The figure shows three views and two pictorial views of one solid part (mm, origin at its lowest corner). Answer the questions. Round coordinates to 2 decimals unless told otherwise and drop trailing zeros. Loops run counter-clockwise (first coordinate to the right, second up) from the corner with the lowest first, then second, coordinate; pieces in that order, holes last. Notation, with made-up numbers: (40.5, 47.25) -> (91.5, 47.25) arc R28 cw to (91.5, 69.25) -> close; hole circle Ø8 at (73.25, 42). An arc over 180 degrees is marked (long way). Use a Markdown table: item, result. Add a question column.
Q1. For a pull along X with two mould halves and no side action, classify the marked faces 1, 2 and 3 as released by +X, released by -X, zero draft, split by the parting line, or undercut.
Q2. Section B-B on z = 2.05 is taken. Give the vertices of the cut face in (x, y).
Q3. Given pin 1 Ø5 at (x, y) = (37.5, 49) entering from -Z; pin 2 Ø12.5 at (x, y) = (38.5, 35.5) entering from +Z; pin 3 Ø12 at (x, y) = (57, 33) entering from +Z; pin 4 Ø1.5 at (y, z) = (47, 1) entering from -X (1 decimal), each flat-ended and moving along its own axis, determine where each tip first touches the part or whether it passes through.
Q4. Consider line 1 (Y direction, x = 40, z = 2.15); line 2 (Y direction, x = 17.5, z = 5.5) (1 decimal); line 3 (X direction, y = 33.5, z = 0.5). Determine where each line is inside the solid, lowest interval first.
Q5. Section A-A on x = 40 is taken. Give the vertices of the cut face in (y, z).
Q6. Section D-D on y = 9 is taken. Give the vertices of the cut face in (x, z) (1 decimal).
Q7. Section C-C on y = 40 is taken. Give the vertices of the cut face in (x, z).
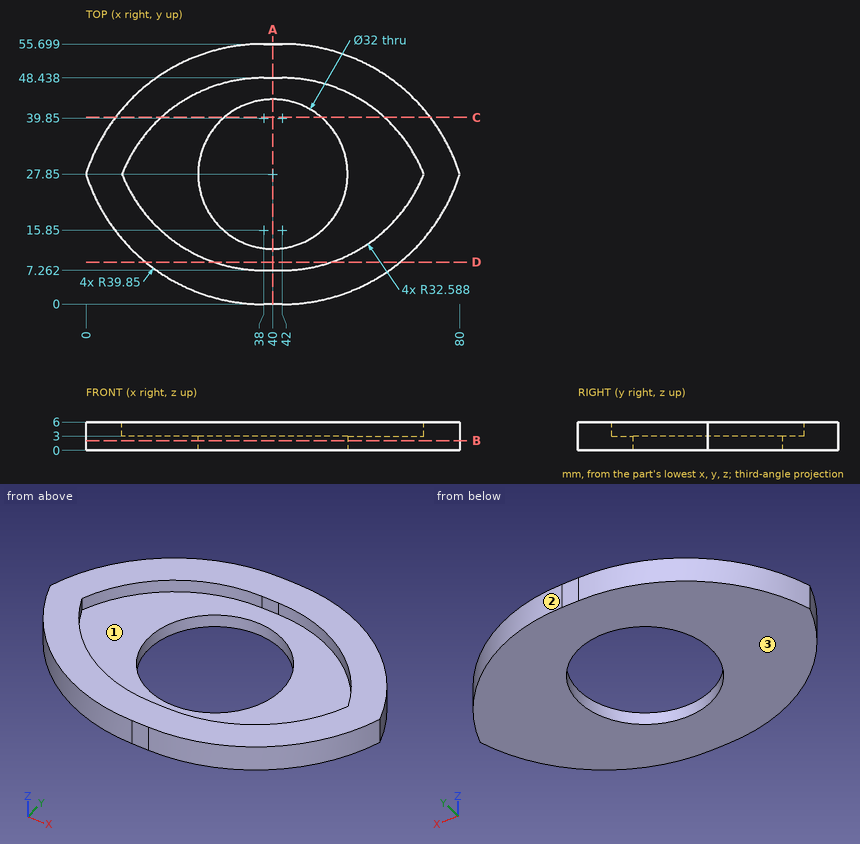
Checked values:
| question | item | result |
|---|---|---|
| 1 | face 1 | undercut |
| 1 | face 2 | released by +X |
| 1 | face 3 | zero draft |
| 2 | outline | (0, 27.85) arc R39.85 ccw to (38, 0) -> (42, 0) arc R39.85 ccw to (80, 27.85) arc R39.85 ccw to (42, 55.7) -> (38, 55.7) arc R39.85 ccw to start; hole circle Ø32 at (40, 27.85) |
| 3 | pin 1 | stops at z = 0 |
| 3 | pin 2 | passes through |
| 3 | pin 3 | stops at z = 3 |
| 3 | pin 4 | stops at x = 12.2 |
| 4 | line 1 | y = 0 to 11.85, 43.85 to 55.7 |
| 4 | line 2 | y = 5.7 to 14.5, 41.2 to 50 |
| 4 | line 3 | x = 2.27 to 25.03, 54.97 to 77.73 |
| 5 | outline | (0, 0) -> (11.85, 0) -> (11.85, 3) -> (7.26, 3) -> (7.26, 6) -> (0, 6) -> close; (43.85, 0) -> (55.7, 0) -> (55.7, 6) -> (48.44, 6) -> (48.44, 3) -> (43.85, 3) -> close |
| 6 | outline | (12.8, 0) -> (67.2, 0) -> (67.2, 6) -> (52.5, 6) -> (52.5, 3) -> (27.5, 3) -> (27.5, 6) -> (12.8, 6) -> close |
| 7 | outline | (6.3, 0) -> (29.59, 0) -> (29.59, 3) -> (16.12, 3) -> (16.12, 6) -> (6.3, 6) -> close; (50.41, 0) -> (73.7, 0) -> (73.7, 6) -> (63.88, 6) -> (63.88, 3) -> (50.41, 3) -> close |
